from build123d import *

# Parameters (mm, degrees)
EXTRUDE_1_DEPTH     = 30
SKETCH_2_R          = 5
CUT_EXTRUDE_1_DEPTH = 71
EXTRUDE_6_DEPTH     = 20
SKETCH_3_7_W        = 4.398
SKETCH_3_7_H        = 10.5
SKETCH_3_7_H_2      = 3.285510203
EXTRUDE_7_DEPTH     = 30
SKETCH_5_W          = 2.915886522
SKETCH_5_H          = 13.785510203
EXTRUDE_8_DEPTH     = 30
SKETCH_6_W          = 7.313886522
SKETCH_6_H          = 15
SKETCH_6_W_2        = 5
EXTRUDE_9_DEPTH     = 10
SKETCH_7_W          = 3.04
SKETCH_7_H          = 13
EXTRUDE_10_DEPTH    = 30
SKETCH_8_W          = 3.04
SKETCH_8_H          = 15
EXTRUDE_11_DEPTH    = 10
SKETCH_10_W         = 2.5
SKETCH_10_H         = 23
SKETCH_10_W_2       = 5.602
SKETCH_10_H_2       = 23.785510203
EXTRUDE_12_DEPTH    = 15
SKETCH_11_W         = 5.602
SKETCH_11_H         = 13.785510203
EXTRUDE_13_DEPTH    = 15
SKETCH_13_W         = 2.5
SKETCH_13_H         = 13
EXTRUDE_14_DEPTH    = 15
FILLET_1_R          = 2
SKETCH_14_W         = 4.252343595
SKETCH_14_H         = 32
CUT_EXTRUDE_2_DEPTH = 12
SKETCH_15_W         = 12
SKETCH_15_H         = 6.952343595
EXTRUDE_15_DEPTH    = 2
FILLET_2_R          = 2
CUT_EXTRUDE_3_DEPTH = 32
SKETCH_17_W         = 12.915886522
SKETCH_17_H         = 7.23748014
EXTRUDE_17_DEPTH    = 2
FILLET_3_R          = 2
SKETCH_20_W         = 10.54
SKETCH_20_H         = 0.8
CUT_EXTRUDE_4_DEPTH = 30
FILLET_5_R          = 2
SKETCH_21_W         = 10.244070675
SKETCH_21_H         = 15
CUT_EXTRUDE_5_DEPTH = 64
CUT_EXTRUDE_6_DEPTH = 64
SKETCH_23_W         = 64
SKETCH_23_H         = 30
EXTRUDE_18_DEPTH    = 2
FILLET_7_R          = 2
EXTRUDE_START       = 20
EXTRUDE_19_DEPTH    = 30


# Read off the part's stored shape, not the designer's step: 凸台-拉伸19
with BuildPart() as part:
    # 草图1 → 凸台-拉伸1 (new body)
    with BuildSketch(Plane.XY):
        Polygon((0, 20), (0, 0), (60, 0), (60, 20), (30, 20), align=None)
    extrude(amount=EXTRUDE_1_DEPTH)

    # 草图2 → 切除-拉伸1 (cut, through all)
    with BuildSketch(Plane.XY.offset(30)):
        with Locations((15, 10)):
            Circle(SKETCH_2_R)
        with Locations((45, 10)):
            Circle(SKETCH_2_R)
    extrude(amount=-CUT_EXTRUDE_1_DEPTH, mode=Mode.SUBTRACT)

    # 草图3 → 凸台-拉伸6 (add)
    with BuildSketch(Plane(origin=(0, 20, 0), x_dir=(1, 0, 0), z_dir=(0, 1, 0))):
        Polygon((60.96, -17), (60.96, -30), (64, -30), (64, 0), (60, 0), (60, -17), align=None)
        Polygon((60, -19.5), (60, -30), (60.96, -30), (60.96, -17), (60, -17), align=None)
    extrude(amount=-EXTRUDE_6_DEPTH)

    # 草图3<7> → 凸台-拉伸7 (add)
    with BuildSketch(Plane(origin=(0, 20, 0), x_dir=(1, 0, 0), z_dir=(0, 1, 0))):
        with Locations((7.801, -24.75)):
            Rectangle(SKETCH_3_7_W, SKETCH_3_7_H)
        with Locations((7.801, -17.857244898)):
            Rectangle(SKETCH_3_7_W, SKETCH_3_7_H_2)
        Polygon((60.96, -17), (60.96, -30), (55.96, -30), (55.96, -17), (58.46, -17), align=None)
    extrude(amount=EXTRUDE_7_DEPTH)

    # 草图5 → 凸台-拉伸8 (add)
    with BuildSketch(Plane(origin=(0, 20, 0), x_dir=(1, 0, 0), z_dir=(0, 1, 0))):
        with Locations((11.457943261, -23.107244899)):
            Rectangle(SKETCH_5_W, SKETCH_5_H)
    extrude(amount=EXTRUDE_8_DEPTH)

    # 草图6 → 凸台-拉伸9 (add)
    with BuildSketch(Plane.XY.offset(30)):
        with Locations((9.258943261, 42.5)):
            Rectangle(SKETCH_6_W, SKETCH_6_H)
        with Locations((58.46, 42.5)):
            Rectangle(SKETCH_6_W_2, SKETCH_6_H)
    extrude(amount=EXTRUDE_9_DEPTH)

    # 草图7 → 凸台-拉伸10 (add)
    with BuildSketch(Plane(origin=(0, 20, 0), x_dir=(1, 0, 0), z_dir=(0, 1, 0))):
        with Locations((62.48, -23.5)):
            Rectangle(SKETCH_7_W, SKETCH_7_H)
    extrude(amount=EXTRUDE_10_DEPTH)

    # 草图8 → 凸台-拉伸11 (add)
    with BuildSketch(Plane.XY.offset(30)):
        with Locations((62.48, 42.5)):
            Rectangle(SKETCH_8_W, SKETCH_8_H)
    extrude(amount=EXTRUDE_11_DEPTH)

    # 草图10 → 凸台-拉伸12 (add)
    with BuildSketch(Plane(origin=(0, 50, 0), x_dir=(1, 0, 0), z_dir=(0, 1, 0))):
        with Locations((54.71, -28.5)):
            Rectangle(SKETCH_10_W, SKETCH_10_H)
        with Locations((2.801, -28.107244898)):
            Rectangle(SKETCH_10_W_2, SKETCH_10_H_2)
    extrude(amount=-EXTRUDE_12_DEPTH)

    # 草图11 → 凸台-拉伸13 (add)
    with BuildSketch(Plane(origin=(0, 20, 0), x_dir=(1, 0, 0), z_dir=(0, 1, 0))):
        with Locations((2.801, -23.107244899)):
            Rectangle(SKETCH_11_W, SKETCH_11_H)
    extrude(amount=EXTRUDE_13_DEPTH)

    # 草图13 → 凸台-拉伸14 (add)
    with BuildSketch(Plane.XZ.offset(-35)):
        with Locations((54.71, 23.5)):
            Rectangle(SKETCH_13_W, SKETCH_13_H)
    extrude(amount=EXTRUDE_14_DEPTH)

    # 圆角1
    fillet_1_edges = [part.edges().sort_by_distance(p)[0] for p in [
        (64, 20, 8.5),
        (64, 35, 17),
        (64, 35, 35),
        (64, 42.5, 40),
        (53.46, 42.5, 40),
        (53.46, 35, 17),
        (0, 42.5, 40),
        (0, 35, 16.214489797),
        (0, 35, 35),
        (0, 20, 8.107244899),
        (53.46, 35, 35),
        (53.46, 27.5, 30),
        (0, 17.5, 30),
        (64, 0, 15),
        (64, 10, 0),
        (64, 17.5, 30),
        (0, 10, 0),
        (32, 0, 30),
        (32, 20, 0),
        (33.187943261, 20, 30),
        (12.915886522, 35, 16.214489797),
        (32, 0, 0),
        (12.915886522, 27.5, 30),
        (12.915886522, 35, 35),
        (12.915886522, 42.5, 40),
        (6.457943261, 50, 40),
        (6.457943261, 35, 40),
        (0, 0, 15),
        (58.73, 35, 40),
        (58.73, 50, 40),
    ]]
    fillet(fillet_1_edges, radius=FILLET_1_R)

    # 草图14 → 切除-拉伸2 (cut)
    with BuildSketch(Plane(origin=(64, 0, 0), x_dir=(0, 0, -1), z_dir=(1, 0, 0))):
        with Locations((-16.873828203, 34)):
            Rectangle(SKETCH_14_W, SKETCH_14_H)
        Polygon((-21.7, 50), (-21.7, 37), (-21.7, 18), (-19, 18), (-19, 50), align=None)
    extrude(amount=-CUT_EXTRUDE_2_DEPTH, mode=Mode.SUBTRACT)

    # 草图15 → 凸台-拉伸15 (add)
    with BuildSketch(Plane(origin=(0, 18, 0), x_dir=(1, 0, 0), z_dir=(0, 1, 0))):
        with Locations((58, -18.223828203)):
            Rectangle(SKETCH_15_W, SKETCH_15_H)
    extrude(amount=EXTRUDE_15_DEPTH)

    # 圆角2
    fillet_2_edges = [part.edges().sort_by_distance(p)[0] for p in [
        (64, 20, 18.223828202),
    ]]
    fillet(fillet_2_edges, radius=FILLET_2_R)

    # 草图16 → 切除-拉伸3 (cut)
    with BuildSketch(Plane(origin=(0, 50, 0), x_dir=(1, 0, 0), z_dir=(0, 1, 0))):
        with BuildLine():
            Line((0, -18.214489797), (0, -22.5))
            Line((0, -22.5), (12.915886522, -22.5))
            Line((12.915886522, -22.5), (12.915886522, -18.214489797))
            ThreePointArc((12.915886522, -18.214489797), (12.330100084, -16.800276235), (10.915886522, -16.214489797))
            Line((10.915886522, -16.214489797), (2, -16.214489797))
            ThreePointArc((2, -16.214489797), (0.585786438, -16.800276235), (0, -18.214489797))
        make_face()
        with BuildLine():
            Line((-1.657142537, -22.5), (0, -22.5))
            Line((0, -22.5), (0, -18.214489797))
            ThreePointArc((0, -18.214489797), (0.585786438, -16.800276235), (2, -16.214489797))
            Line((2, -16.214489797), (10.915886522, -16.214489797))
            ThreePointArc((10.915886522, -16.214489797), (12.330100084, -16.800276235), (12.915886522, -18.214489797))
            Line((12.915886522, -18.214489797), (12.915886522, -15.26251986))
            Line((12.915886522, -15.26251986), (-1.657142537, -15.26251986))
            Line((-1.657142537, -15.26251986), (-1.657142537, -22.5))
        make_face()
    extrude(amount=-CUT_EXTRUDE_3_DEPTH, mode=Mode.SUBTRACT)

    # 草图17 → 凸台-拉伸17 (add)
    with BuildSketch(Plane(origin=(0, 18, 0), x_dir=(1, 0, 0), z_dir=(0, 1, 0))):
        with Locations((6.457943261, -18.88125993)):
            Rectangle(SKETCH_17_W, SKETCH_17_H)
    extrude(amount=EXTRUDE_17_DEPTH)

    # 圆角3
    fillet_3_edges = [part.edges().sort_by_distance(p)[0] for p in [
        (0, 20, 18.88125993),
    ]]
    fillet(fillet_3_edges, radius=FILLET_3_R)

    # 草图20 → 切除-拉伸4 (cut)
    with BuildSketch(Plane(origin=(0, 50, 0), x_dir=(1, 0, 0), z_dir=(0, 1, 0))):
        with Locations((58.73, -22.1)):
            Rectangle(SKETCH_20_W, SKETCH_20_H)
    extrude(amount=-CUT_EXTRUDE_4_DEPTH, mode=Mode.SUBTRACT)

    # 圆角5
    fillet_5_edges = [part.edges().sort_by_distance(p)[0] for p in [
        (64, 20, 22.1),
    ]]
    fillet(fillet_5_edges, radius=FILLET_5_R - 0.0001)  # a hair under: the kernel refuses the full size

    # 草图21 → 切除-拉伸5 (cut)
    with BuildSketch(Plane.ZY):
        with Locations((35.122035338, 42.5)):
            Rectangle(SKETCH_21_W, SKETCH_21_H)
    extrude(amount=-CUT_EXTRUDE_5_DEPTH, mode=Mode.SUBTRACT)

    # 草图22 → 切除-拉伸6 (cut)
    with BuildSketch(Plane.XY.offset(30)):
        with BuildLine():
            Line((56.5, 20), (56.5, 37))
            Line((56.5, 37), (56.5, 50))
            Line((56.5, 50), (53.46, 50))
            Line((53.46, 50), (53.46, 37))
            ThreePointArc((53.46, 37), (54.045786438, 35.585786438), (55.46, 35))
            Line((55.46, 35), (55.46, 20))
            Line((55.46, 20), (56.5, 20))
        make_face()
        with BuildLine():
            Line((53.46, 20), (55.46, 20))
            Line((55.46, 20), (55.46, 35))
            ThreePointArc((55.46, 35), (54.045786438, 35.585786438), (53.46, 37))
            Line((53.46, 37), (53.46, 20))
        make_face()
    extrude(amount=-CUT_EXTRUDE_6_DEPTH, mode=Mode.SUBTRACT)

    # 草图23 → 凸台-拉伸18 (add)
    with BuildSketch(Plane(origin=(0, 20, 0), x_dir=(1, 0, 0), z_dir=(0, 1, 0))):
        with Locations((32, -15)):
            Rectangle(SKETCH_23_W, SKETCH_23_H)
    extrude(amount=-EXTRUDE_18_DEPTH)

    # 圆角7
    fillet_7_edges = [part.edges().sort_by_distance(p)[0] for p in [
        (0, 19, 0),
        (64, 19, 0),
        (64, 19, 30),
        (0, 19, 30),
    ]]
    fillet(fillet_7_edges, radius=FILLET_7_R)

    # 凸台-拉伸19 outline → 凸台-拉伸19 (add)
    with BuildSketch(Plane(origin=(0, 0, 0), x_dir=(1, 0, 0), z_dir=(0, 1, 0)).offset(EXTRUDE_START)):
        with BuildLine():
            Line((14, -30), (14, -22.5))
            Line((14, -22.5), (12.915886522, -22.5))
            Line((12.915886522, -22.5), (12.915886522, -28))
            ThreePointArc((12.915886522, -28), (12.330100084, -29.414213562), (10.915886522, -30))
            Line((10.915886522, -30), (14, -30))
        make_face()
        with BuildLine():
            ThreePointArc((2, -30), (0.585786438, -29.414213562), (0, -28))
            Line((0, -28), (0, -30))
            Line((0, -30), (2, -30))
        make_face()
    extrude(amount=EXTRUDE_19_DEPTH)


solid = part.part
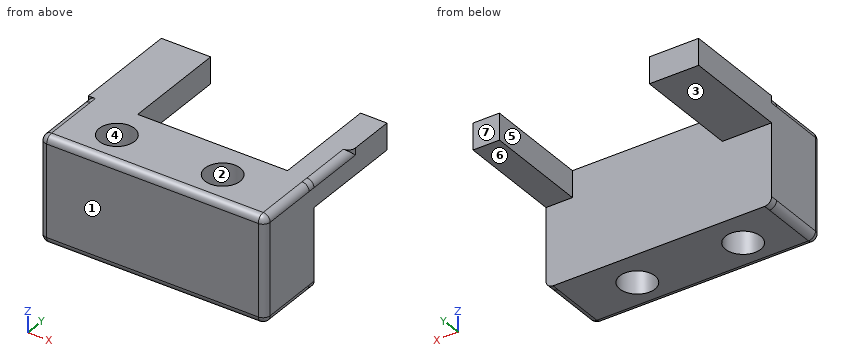
Here's how the part is built. I have some questions about the finished solid (model axes, mm). Face numbers are marked on the shaded views. A direction names the side the tool comes from. Coordinates: 2 decimals unless noted, no trailing zeros. Write each loop counter-clockwise with the first axis right and the second up, starting at its lowest first coordinate (ties: lowest second). Pieces come first, ordered by that corner, then holes.
Item 1: I want a section at C-C on x = 45. Write out the boundary of the cut face in (y, z), and give its area (3 significant figures).
Item 2: I want a section at B-B on y = 21. Write out the boundary of the cut face in (x, z), and give its area (3 significant figures).
Item 3: On a 3-axis mill with a long thin cutter (end or side, diameter ignored), from which of +Z, -Z, +X, -X, +Y, -Y can I reach the whole of each face in a straight line? I mean the marked faces 5, 6 and 7. Say none if no direction works.
Item 4: I want a section at A-A on z = 24. Write out the boundary of the cut face in (x, y).
Item 5: If I drill on line 1 (Y direction, x = 15, z = 6); line 2 (X direction, y = 6.5, z = 20); line 3 (X direction, y = 10.5, z = 2), over which ranges is the centre line in solid material (lowest first)?
Item 6: If we mould it in two halves opening along Y, with no side actions, what happens to the marked faces 1, 2, 3 and 4? For each: +Y half, -Y half, draft (parallel to the pull), parting line (faces both ways), or undercut.
Item 7: I want a section at D-D on y = 10. Write out the boundary of the cut face in (x, z), and give its area (3 significant figures).
Item 8: Will these pins go through, and if not, where does the flat tip stop? pin 1 (6 mm diameter, centred on x = 45, y = 10, fed in from +Z); pin 2 (1 mm diameter, centred on x = 1, z = 1, fed in from -Y); pin 3 (0.6 mm diameter, centred on x = 1, z = 29.5, fed in from -Y); pin 4 (9 mm diameter, centred on x = 20, z = 14, fed in from +Y).
Findings below:
1. outline: (0, 2) arc R2 ccw to (2, 0) - (5, 0) - (5, 30) - (2, 30) arc R2 ccw to (0, 28) - close; (15, 0) - (20, 0) - (20, 30) - (15, 30) - close
1. area: 298 mm2
2. outline: (0, 22.5) - (14, 22.5) - (14, 30) - (0, 30) - close; (56.5, 22.5) - (64, 22.5) - (64, 28) arc R2 ccw to (62, 30) - (56.5, 30) - close
2. area: 160 mm2
3. face 5: +Z, -Z, +Y
3. face 6: -Z, +X, -X, +Y
3. face 7: +Z, -Z, +X, -X, +Y
4. outline: (0, 2) arc R2 ccw to (2, 0) - (62, 0) arc R2 ccw to (64, 2) - (64, 50) - (56.5, 50) - (56.5, 20) - (14, 20) - (14, 50) - (0, 50) - close; hole circle Ø10 at (15, 10); hole circle Ø10 at (45, 10)
5. line 1: y = 0 to 5, 15 to 20
5. line 2: x = 0 to 11.43, 18.57 to 41.43, 48.57 to 64
5. line 3: x = 0 to 10.03, 19.97 to 40.03, 49.97 to 64
6. face 1: -Y half
6. face 2: undercut
6. face 3: draft
6. face 4: undercut
7. outline: (0, 2) arc R2 ccw to (2, 0) - (10, 0) - (10, 30) - (2, 30) arc R2 ccw to (0, 28) - close; (20, 0) - (40, 0) - (40, 30) - (20, 30) - close; (50, 0) - (62, 0) arc R2 ccw to (64, 2) - (64, 28) arc R2 ccw to (62, 30) - (50, 30) - close
7. area: 1,320 mm2
8. pin 1: passes through
8. pin 2: stops at y = 0.22
8. pin 3: stops at y = 0.68
8. pin 4: stops at y = 20
